```python
from build123d import *

# Parameters (mm, degrees)
F1_DEPTH     = 10.16
F2_W         = 3.81
F2_H         = 3.81
F3_DEPTH     = 25.4
F4_R         = 1.5875
F5_T4_DEPTH  = 20.32
F5_T10_DEPTH = 20.32
F5_T16_DEPTH = 20.32
F5_T23_DEPTH = 20.32
F5_T29_DEPTH = 20.32
F6_SIZE      = 3.175
F7_SIZE      = 0.762
F8_SIZE      = 0.762
F10_D        = 1.778
F12_DEPTH    = 25.4


# Not quite as in the source:
# - a fillet or chamfer that OpenCascade refuses, or shapes differently, is made with other operations: its cross-section is extruded or revolved along the edge and cut away or added


with BuildPart() as f1:
    # F0 (on Front) → F1 (new body, symmetric)
    with BuildSketch(Plane.XZ):
        Polygon((-8.382, 0), (-0.4445, 0), (-1.1748426721, -2.0066), (5.1751573279, -2.0066), (4.4448146558, 0), (15.24, 0), (15.24, 1.778), (-3.81, 1.778), (-3.81, 6.6675), (-10.16, 6.6675), (-10.16, -4.7625), (-8.382, -4.7625), align=None)
    extrude(amount=F1_DEPTH, both=True)

    # F2 (on face) → F3 (cut)
    with BuildSketch(Plane(origin=(-10.16, 0, 0), x_dir=(0, -1, 0), z_dir=(-1, 0, 0))):
        with Locations((0, 4.7625)):
            Rectangle(F2_W, F2_H)
    extrude(amount=-F3_DEPTH, mode=Mode.SUBTRACT)

    # F4
    f4_edges = [f1.edges().sort_by_distance(p)[0] for p in [
        (-8.382, 0, 0),
    ]]
    fillet(f4_edges, radius=F4_R)

    # F5: fillet of radius 3.81 on 1 edges, made by hand


with BuildPart() as f5_tool2:
    # F5_s3 → F5_t4 (new body)
    with BuildSketch(Plane.XZ.offset(10.16)):
        with BuildLine():
            ThreePointArc((-3.81, 5.588), (-2.6940768363, 2.8939231637), (0, 1.778))
            Line((0, 1.778), (-3.81, 1.778))
            Line((-3.81, 1.778), (-3.81, 5.588))
        make_face()
    extrude(amount=-F5_T4_DEPTH)

    split(bisect_by=Plane.XZ.offset(1.905), keep=Keep.TOP)

    split(bisect_by=Plane.XY.offset(2.8575), keep=Keep.TOP)


with BuildPart() as f1_1:
    add(f1.part)

    # F5_t1: union F5_tool2
    add(f5_tool2.part)


with BuildPart() as f5_tool8:
    # F5_s9 → F5_t10 (new body)
    with BuildSketch(Plane.XZ.offset(10.16)):
        with BuildLine():
            ThreePointArc((-3.81, 5.588), (-2.6940768363, 2.8939231637), (0, 1.778))
            Line((0, 1.778), (-3.81, 1.778))
            Line((-3.81, 1.778), (-3.81, 5.588))
        make_face()
    extrude(amount=-F5_T10_DEPTH)

    split(bisect_by=Plane.XZ.offset(1.905), keep=Keep.TOP)

    split(bisect_by=Plane.XY.offset(2.8575), keep=Keep.BOTTOM)


with BuildPart() as f1_2:
    add(f1_1.part)

    # F5_t7: union F5_tool8
    add(f5_tool8.part)


with BuildPart() as f5_tool14:
    # F5_s15 → F5_t16 (new body)
    with BuildSketch(Plane.XZ.offset(10.16)):
        with BuildLine():
            ThreePointArc((-3.81, 5.588), (-2.6940768363, 2.8939231637), (0, 1.778))
            Line((0, 1.778), (-3.81, 1.778))
            Line((-3.81, 1.778), (-3.81, 5.588))
        make_face()
    extrude(amount=-F5_T16_DEPTH)

    split(bisect_by=Plane.XZ.offset(1.905), keep=Keep.BOTTOM)

    split(bisect_by=Plane.XY.offset(2.8575), keep=Keep.BOTTOM)

    split(bisect_by=Plane.XZ.offset(-1.905), keep=Keep.TOP)


with BuildPart() as f1_3:
    add(f1_2.part)

    # F5_t13: union F5_tool14
    add(f5_tool14.part)


with BuildPart() as f5_tool21:
    # F5_s22 → F5_t23 (new body)
    with BuildSketch(Plane.XZ.offset(10.16)):
        with BuildLine():
            ThreePointArc((-3.81, 5.588), (-2.6940768363, 2.8939231637), (0, 1.778))
            Line((0, 1.778), (-3.81, 1.778))
            Line((-3.81, 1.778), (-3.81, 5.588))
        make_face()
    extrude(amount=-F5_T23_DEPTH)

    split(bisect_by=Plane.XY.offset(2.8575), keep=Keep.TOP)

    split(bisect_by=Plane.XZ.offset(-1.905), keep=Keep.BOTTOM)


with BuildPart() as f1_4:
    add(f1_3.part)

    # F5_t20: union F5_tool21
    add(f5_tool21.part)


with BuildPart() as f5_tool27:
    # F5_s28 → F5_t29 (new body)
    with BuildSketch(Plane.XZ.offset(10.16)):
        with BuildLine():
            ThreePointArc((-3.81, 5.588), (-2.6940768363, 2.8939231637), (0, 1.778))
            Line((0, 1.778), (-3.81, 1.778))
            Line((-3.81, 1.778), (-3.81, 5.588))
        make_face()
    extrude(amount=-F5_T29_DEPTH)

    split(bisect_by=Plane.XY.offset(2.8575), keep=Keep.BOTTOM)

    split(bisect_by=Plane.XZ.offset(-1.905), keep=Keep.BOTTOM)


with BuildPart() as f1_5:
    add(f1_4.part)

    # F5_t26: union F5_tool27
    add(f5_tool27.part)

    # F6
    f6_edges = [f1_5.edges().sort_by_distance(p)[0] for p in [
        (-3.509976, -1.905, 4.106052),
        (-3.509976, 1.905, 4.106052),
    ]]
    chamfer(f6_edges, length=F6_SIZE)

    # F7
    f7_edges = [f1_5.edges().sort_by_distance(p)[0] for p in [
        (-10.16, 0, -4.7625),
    ]]
    chamfer(f7_edges, length=F7_SIZE)

    # F8
    f8_edges = [f1_5.edges().sort_by_distance(p)[0] for p in [
        (-2.694077, -10.16, 2.893923),
        (7.62, -10.16, 1.778),
        (7.62, 10.16, 1.778),
        (15.24, 0, 1.778),
    ]]
    chamfer(f8_edges, length=F8_SIZE)

    # F10 (through all)
    with Locations(Plane(origin=(0, 0, -2.0066), x_dir=(1, 0, 0), z_dir=(0, 0, -1))):
        with Locations((2.0001573279, 3.81), (2.0001573279, -3.81)):
            Hole(F10_D / 2)

    # F11 (on face) → F12 (cut)
    with BuildSketch(Plane.XZ.offset(10.16)):
        Polygon((-10.16, -3.4925), (-10.16, -4.0005), (-9.7200590949, -3.7465), align=None)
        Polygon((-10.16, -2.9845), (-10.16, -3.4925), (-9.7200590949, -3.2385), align=None)
        Polygon((-10.16, -2.4765), (-10.16, -2.9845), (-9.7200590949, -2.7305), align=None)
        Polygon((-9.7200590949, -2.2225), (-10.16, -1.9685), (-10.16, -2.4765), align=None)
        Polygon((-9.7200590949, -1.7145), (-10.16, -1.4605), (-10.16, -1.9685), align=None)
        Polygon((-9.7200590949, -1.2065), (-10.16, -0.9525), (-10.16, -1.4605), align=None)
        Polygon((-9.7200590949, -0.6985), (-10.16, -0.4445), (-10.16, -0.9525), align=None)
        Polygon((-9.7200590949, -0.1905), (-10.16, 0.0635), (-10.16, -0.4445), align=None)
        Polygon((-9.7200590949, 0.3175), (-10.16, 0.5715), (-10.16, 0.0635), align=None)
        Polygon((-9.7200590949, 0.8255), (-10.16, 1.0795), (-10.16, 0.5715), align=None)
        Polygon((-9.7200590949, 1.3335), (-10.16, 1.5875), (-10.16, 1.0795), align=None)
        Polygon((-9.7200590949, 1.8415), (-10.16, 2.0955), (-10.16, 1.5875), align=None)
        Polygon((-9.7200590949, 2.3495), (-10.16, 2.6035), (-10.16, 2.0955), align=None)
        Polygon((-9.7200590949, 2.8575), (-10.16, 3.1115), (-10.16, 2.6035), align=None)
        Polygon((-9.7200590949, 3.3655), (-10.16, 3.6195), (-10.16, 3.1115), align=None)
        Polygon((-9.7200590949, 3.8735), (-10.16, 4.1275), (-10.16, 3.6195), align=None)
        Polygon((-9.7200590949, 4.3815), (-10.16, 4.6355), (-10.16, 4.1275), align=None)
        Polygon((-9.7200590949, 4.8895), (-10.16, 5.1435), (-10.16, 4.6355), align=None)
        Polygon((-9.7200590949, 5.3975), (-10.16, 5.6515), (-10.16, 5.1435), align=None)
        Polygon((-9.7200590949, 5.9055), (-10.16, 6.1595), (-10.16, 5.6515), align=None)
        Polygon((-10.16, 6.1595), (-9.7200590949, 6.4135), (-10.16, 6.6675), align=None)
    extrude(amount=-F12_DEPTH, mode=Mode.SUBTRACT)


solid = f1_5.part
```
Design review of the part built by this model. Coordinates are the model's own, in mm. A direction names the side the tool comes from. Round coordinates to 2 decimals unless told otherwise and drop trailing zeros. Write each loop counter-clockwise with the first axis right and the second up, starting at its lowest first coordinate (ties: lowest second). Pieces come first, ordered by that corner, then holes. Notation, with made-up numbers: (79.25, 52.25) -> (95.25, 52.25) arc R23 ccw to (95.25, 64.25) -> close; hole circle Ø7 at (10.25, 71). An arc over 180 degrees is marked (long way). Write item = value, one per line. Start each with the question number.
1) Take a section at A-A, the plane x = 6.5. State the section outline as (y, z) points.
2) Wall thickness on probe 1 along Y at (x, z) = (-7.25, 5.75) (3 decimals); probe 2 along X at (y, z) = (-3.81, -1.1); probe 3 along Z at (x, y) = (8.5, 3): over which ranges is each line inside the solid? List them lowest first. Write a range as from..to.
3) Mouldability with a two-part tool opening along Z and no side actions: class faces 1 (the face through (2.655, 3.209, -0.088)), 2 (the face through (-4.833, 3.823, 4.066)), 3 (the face through (-0.805, -0.142, -0.989)) as +Z half, -Z half, draft (parallel to the pull), parting line (faces both ways), or undercut.
4) Take a section at B-B, the plane x = 1.75. State the section outline as (y, z) points.
5) Tool access review of faces 4 (the face through (-8, 1.905, 5)), 5 (the face through (-5, 0, 2.858)), 6 (the face through (-3.81, -7, 6)), 7 (the face through (-7.9, 0.14, -0.45)): name each direction out of +Z, -Z, +X, -X, +Y, -Y from which nothing blocks a thin tool from reaching the whole face with its end or side.
6) Clearance check with flat-ended pins moving along their axes: pin 1 (0.5 mm diameter, centred on y = -7.5, z = 6, fed in from +X); pin 2 (7 mm diameter, centred on x = -3.5, y = 3.5, fed in from -Z); pin 3 (5.5 mm diameter, centred on x = 10, y = 4, fed in from -Z); pin 4 (1.6 mm diameter, centred on x = 2, y = 3.81, fed in from -Z). State where each tip first meets the part, or that it passes through.
Results list:
q1.outline = (-10.16, 0) -> (10.16, 0) -> (10.16, 1.02) -> (9.4, 1.78) -> (-9.4, 1.78) -> (-10.16, 1.02) -> close
q2.probe_1 = -10.16..-1.905, 1.905..10.16
q2.probe_2 = -9.9..-8.31, -0.84..1.11, 2.89..4.85
q2.probe_3 = 0..1.78
q3.face_1 = draft
q3.face_2 = +Z half
q3.face_3 = undercut
q4.outline = (-10.16, -2.01) -> (-4.66, -2.01) -> (-4.66, 1.78) -> (-9.4, 1.78) -> (-10.16, 1.02) -> close; (-2.96, -2.01) -> (2.96, -2.01) -> (2.96, 1.78) -> (-2.96, 1.78) -> close; (4.66, -2.01) -> (10.16, -2.01) -> (10.16, 1.02) -> (9.4, 1.78) -> (4.66, 1.78) -> close
q5.face_4 = +Z, +X, -X
q5.face_5 = +Z, +X
q5.face_6 = +Z, +X, +Y, -Y
q5.face_7 = -Z, +Y, -Y
q6.pin_1 = -3.81
q6.pin_2 = -2.01
q6.pin_3 = 0
q6.pin_4 = through
